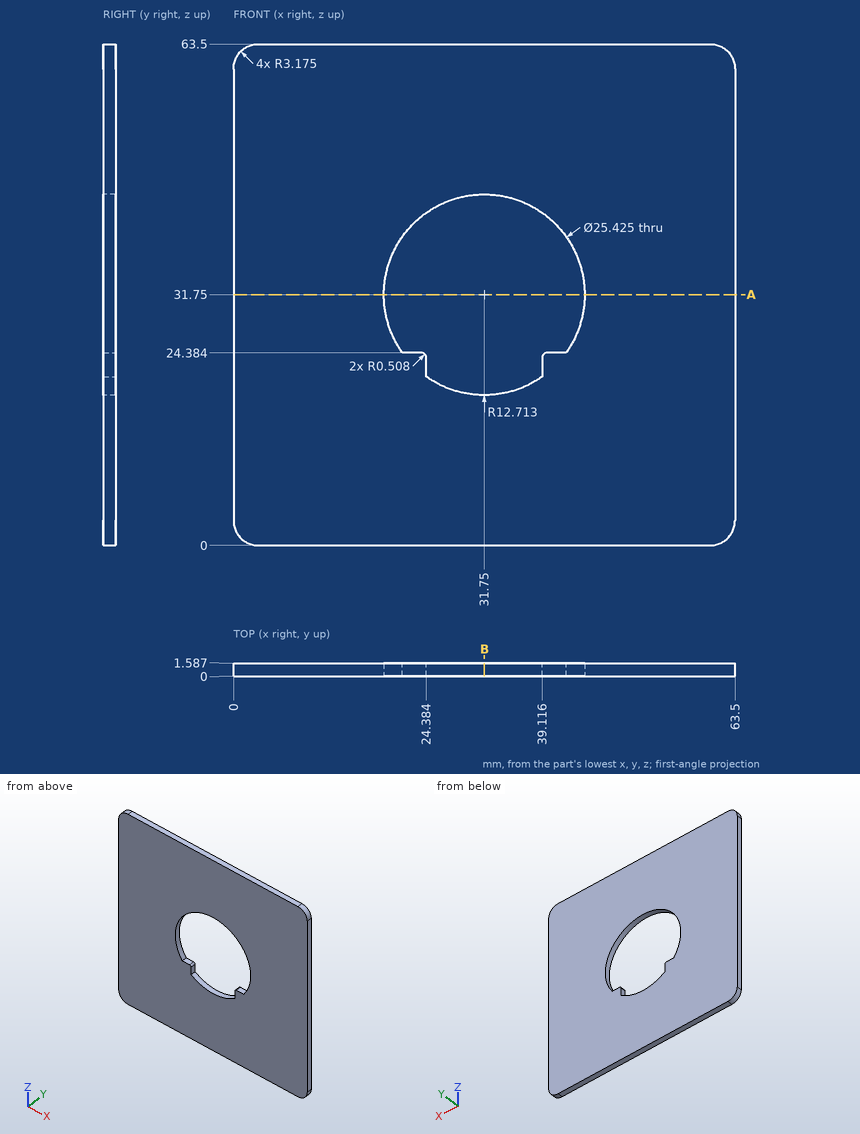
For this review, use the dimensioned drawing (mm, ordinates from the lowest corner) and the shaded views. Round coordinates to 2 decimals unless told otherwise and drop trailing zeros. Write each loop counter-clockwise with the first axis right and the second up, starting at its lowest first coordinate (ties: lowest second). Pieces come first, ordered by that corner, then holes. Notation, with made-up numbers: (60, -26) - (113, -26) arc R15 ccw to (113, -12) - close; hole circle Ø7 at (32.5, -30.75). An arc over 180 degrees is marked (long way). One line per item, written item: value. Start each with the question number.
1. Consider section A-A on z = 31.75. Write out the cut boundary in (x, y).
2. To check wall thickness, follow L1, parallel to X at y = 0.4, z = 31.75; L2, parallel to Z at x = 30, y = 0.9; L3, parallel to X at y = 0.85, z = 34. State the ranges of each line that lie inside material, in increasing order. Write a range as from..to.
3. Consider section B-B on x = 31.75. Write out the cut boundary in (y, z).
Checks:
1. outline: (0, 0) - (19.04, 0) - (19.04, 1.59) - (0, 1.59) - close; (44.46, 0) - (63.5, 0) - (63.5, 1.59) - (44.46, 1.59) - close
2. L1: x = 0..19.04, 44.46..63.5
2. L2: z = 0..19.16, 44.34..63.5
2. L3: x = 0..19.24, 44.26..63.5
3. outline: (0, 0) - (1.59, 0) - (1.59, 19.04) - (0, 19.04) - close; (0, 44.46) - (1.59, 44.46) - (1.59, 63.5) - (0, 63.5) - close
